Design review of the part shown in the three views and the two pictorial views. Dimensions are in mm from the part's minimum x, y and z. A direction names the side the tool comes from. Coordinates: 2 decimals unless noted, no trailing zeros. Write each loop counter-clockwise with the first axis right and the second up, starting at its lowest first coordinate (ties: lowest second). Pieces come first, ordered by that corner, then holes. Notation, with made-up numbers: (3, 19) - (15, 19) arc R27 ccw to (15, 44) - close; hole circle Ø5 at (75, 77). An arc over 180 degrees is marked (long way). Answer as CSV lines item,"result". Start each with the question number.
Q1. We need section C-C (x = 27). Write out the cut boundary in (y, z) (1 decimal), plus the area to 3 significant figures.
Q2. Machinability: for the marked faces 4, 5, 6 and 7, which of the approach directions +Z, -Z, +X, -X, +Y, -Y give a long, thin tool a straight path to every point of the face, cutting with its end or side? Answer none if there is none.
Q3. For line 1 along X through (y, z) = (8.5, 31); line 2 along Z through (x, y) = (18, 11); line 3 along X through (y, z) = (22, 14.5) (1 decimal), list the stretches that pass through material, from the lowest coordinate up. Write a range as [from, to].
Q4. We need section D-D (z = 43). Write out the cut boundary in (x, y) (1 decimal), plus the area to 3 significant figures.
Q5. Clearance check with flat-ended pins moving along their axes: pin 1 (5 mm diameter, centred on y = 30.5, z = 9.5, fed in from -X); pin 2 (7.5 mm diameter, centred on x = 17, y = 30.5, fed in from +Z); pin 3 (11.5 mm diameter, centred on x = 3.5, z = 29, fed in from +Y). State where each tip first meets the part, or that it passes through.
Q6. We need section B-B (y = 30). State how many separate pieces and enclosed holes the cut face has, plus the area to 3 significant figures.
Q7. We need section A-A (z = 3.5). Write out the cut boundary in (x, y), plus the area to 3 significant figures.
Q8. Mouldability with a two-part tool opening along X and no side actions: class the marked faces 1, 2 and 3 as pulls with the +X half, pulls with the -X half, needs draft (parallel to the pull), parting line crosses it, or undercut.
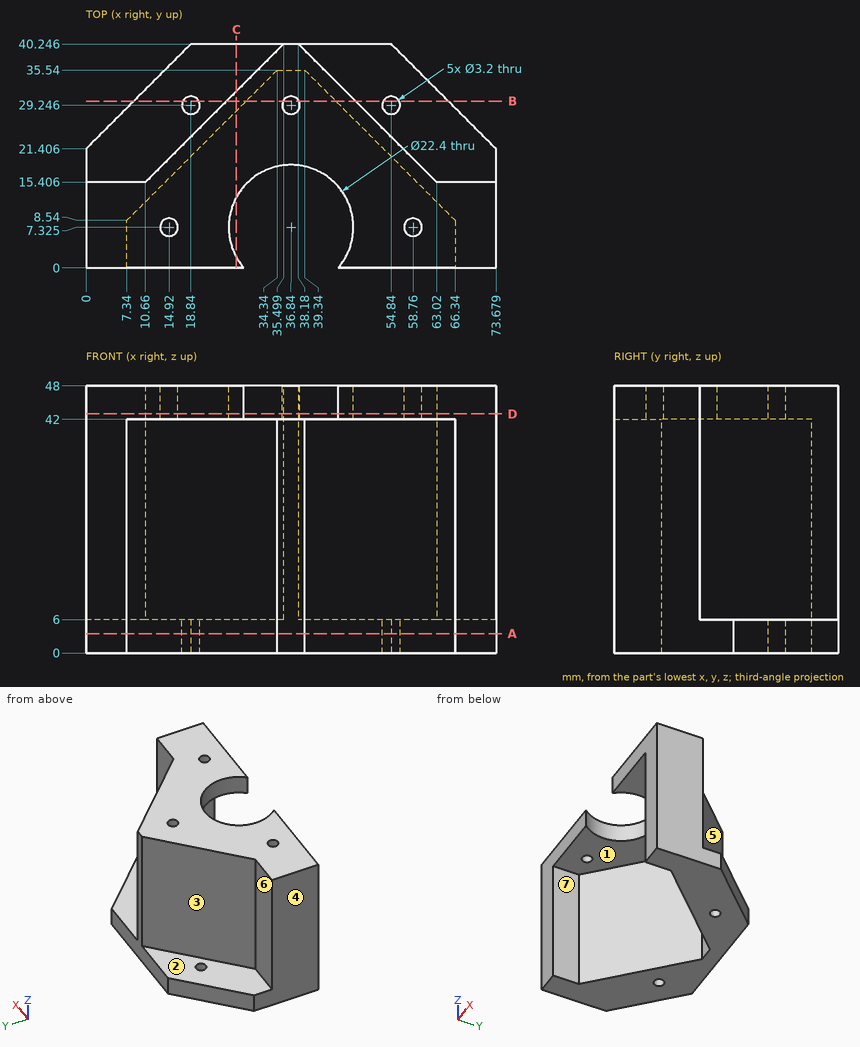
Results list:
1,outline,"(0, 42) - (2, 42) - (2, 48) - (0, 48) - close; (12.7, 42) - (28.2, 42) - (28.2, 0) - (40.2, 0) - (40.2, 6) - (31.7, 6) - (31.7, 48) - (12.7, 48) - close"
1,area,"326 mm2"
2,face 4,"+Z, -Z, -X, +Y, -Y"
2,face 5,"+Z, +X, +Y"
2,face 6,"+Z, -X, +Y"
2,face 7,"-Z, -Y"
3,line 1,"x = [0, 7.34], [66.34, 73.68]"
3,line 2,"z = [42, 48]"
3,line 3,"x = [17.3, 20.8], [52.9, 56.4]"
4,outline,"(0, 0) - (28.4, 0) arc R11.2 cw (long way) to (45.3, 0) - (73.7, 0) - (73.7, 15.4) - (63, 15.4) - (38.2, 40.2) - (35.5, 40.2) - (10.7, 15.4) - (0, 15.4) - close; hole circle Ø3.2 at (14.9, 7.3); hole circle Ø3.2 at (36.8, 29.2); hole circle Ø3.2 at (58.8, 7.3)"
4,area,"1,450 mm2"
5,pin 1,"stops at x = 23.25"
5,pin 2,"stops at z = 6"
5,pin 3,"stops at y = 15.41"
6,separate pieces,"4"
6,enclosed holes,"0"
6,area,"586 mm2"
7,outline,"(0, 0) - (7.34, 0) - (7.34, 8.54) - (34.34, 35.54) - (39.34, 35.54) - (66.34, 8.54) - (66.34, 0) - (73.68, 0) - (73.68, 21.41) - (54.84, 40.25) - (18.84, 40.25) - (0, 21.41) - close; hole circle Ø3.2 at (18.84, 29.25); hole circle Ø3.2 at (54.84, 29.25)"
7,area,"1,230 mm2"
8,face 1,"undercut"
8,face 2,"needs draft"
8,face 3,"pulls with the -X half"
